Autodesk Inventor part; units mm, degrees
ref_plane "YZ Plane" through (0, 0, 0) normal (1, 0, 0) x (0, 1, 0)
ref_plane "XZ Plane" through (0, 0, 0) normal (0, 1, 0) x (-1, 0, 0)
ref_plane "XY Plane" through (0, 0, 0) normal (0, 0, 1) x (1, 0, 0)
sketch "Sketch1" plane through (0, 0, 0) normal (0, 0, 1) x (1, 0, 0)
  line L0 (0, 0) -> (298.0905, 0) construction
  line L1 (381, 254) -> (0, 254)
  line L2 (0, 254) -> (0, 0) construction
  line L3 (0, 254) -> (0, 0) construction
  line L4 (381, 254) -> (381, 177.8)
  line L5 (381, 177.8) -> (298.0905, 0)
  line L6 (0, 254) -> (0, 177.8)
  line L7 (82.9095, 0) -> (0, 177.8)
  line L8 (82.9095, 0) -> (298.0905, 0)
  dimension "d42" = 254
  dimension "d79" = 381
  dimension "d97" = 65
  dimension "d98" = 76.2
  dimension "d99" = 25
extrude "Plate1" add sketch "Sketch1" along normal blind 9.525
fillet "Corner Round1" radius 12.7 2 edges at (298.0905, 0, 4.7625) (82.9095, 0, 4.7625)
ref_plane "Work Plane1" through (0, 177.8, -13.208) normal (0, 1, 0) x (1, 0, 0)
sketch "Sketch10" plane through (0, 177.8, 9.525) normal (0, 0, 1) x (1, 0, 0)
  line L0 (342.9, 53.975) -> (342.9, 47.625) construction
  line L1 (333.375, 53.975) -> (333.375, 47.625)
  line L2 (352.425, 47.625) -> (352.425, 53.975)
  arc A0 (352.425, 53.975) -> (333.375, 53.975) centre (342.9, 53.975) ccw
  arc A1 (333.375, 47.625) -> (352.425, 47.625) centre (342.9, 47.625) ccw
  line L3 (50.8, 53.975) -> (50.8, 47.625) construction
  line L4 (41.275, 53.975) -> (41.275, 47.625)
  line L5 (60.325, 47.625) -> (60.325, 53.975)
  arc A2 (60.325, 53.975) -> (41.275, 53.975) centre (50.8, 53.975) ccw
  arc A3 (41.275, 47.625) -> (60.325, 47.625) centre (50.8, 47.625) ccw
  line L6 (0, 76.2) -> (381, 76.2)
  line L7 (381, 76.2) -> (381, 0)
  arc A4 (282.575, 47.625) -> (301.625, 47.625) centre (292.1, 47.625) ccw
  line L8 (282.575, 53.975) -> (282.575, 47.625)
  arc A5 (301.625, 53.975) -> (282.575, 53.975) centre (292.1, 53.975) ccw
  line L9 (301.625, 47.625) -> (301.625, 53.975)
  arc A6 (187.325, 53.975) -> (168.275, 53.975) centre (177.8, 53.975) ccw
  line L10 (187.325, 47.625) -> (187.325, 53.975)
  arc A7 (168.275, 47.625) -> (187.325, 47.625) centre (177.8, 47.625) ccw
  line L11 (168.275, 53.975) -> (168.275, 47.625)
  line L12 (0, 0) -> (0, 76.2)
  point P0 (342.9, 50.8)
  point P1 (50.8, 50.8)
  point P2 (41.275, 50.8)
  point P3 (168.275, 50.8)
  dimension "d83" = 19.05
  dimension "d85" = 6.35
  dimension "d100" = 25.4
  dimension "d101" = 38.1
  dimension "d104" = 50.8
  dimension "d111" = 127
  dimension "d116" = 50.8
extrude "Cut4" cut sketch "Sketch10" against normal blind 9.525
sketch "Sketch11" plane through (0, 0, 9.525) normal (0, 0, 1) x (1, 0, 0)
  line L0 (165.1, 127) -> (241.3, 127)
  line L1 (254, 114.3) -> (254, 38.1)
  line L2 (241.3, 25.4) -> (165.1, 25.4)
  line L3 (152.4, 38.1) -> (152.4, 114.3)
  line L4 (152.4, 127) -> (254, 25.4) construction
  line L5 (254, 127) -> (152.4, 25.4) construction
  arc A0 (254, 114.3) -> (241.3, 127) centre (241.3, 114.3) ccw
  arc A1 (165.1, 127) -> (152.4, 114.3) centre (165.1, 114.3) ccw
  arc A2 (152.4, 38.1) -> (165.1, 25.4) centre (165.1, 38.1) ccw
  arc A3 (241.3, 25.4) -> (254, 38.1) centre (241.3, 38.1) ccw
  line L6 (289.9997, 0) -> (0, 0)
  line L7 (0, 0) -> (0, 254)
  point P0 (203.2, 76.2)
  point P1 (12.7, 0)
  point P2 (0, 12.7)
  point P3 (0, 155.067)
  dimension "d90" = 101.6
  dimension "d91" = 101.6
  dimension "d92" = 12.7
  dimension "d93" = 25.4
  dimension "d94" = 152.4
extrude "Cut5" cut sketch "Sketch11" against normal blind 9.525
fillet "Corner Round4" radius 6.35 4 edges at (381, 254, 4.7625) (381, 177.8, 4.7625) (0, 254, 4.7625) (0, 177.8, 4.7625)
equation "\"d88\" = Thickness"
equation "\"d95\" = Thickness"
equation "\"d15\" = Thickness"
equation "\"BendReliefWidth\" = Thickness"
equation "\"BendReliefDepth\" = 0.5 * Thickness"
equation "\"CornerReliefSize\" = 4 * Thickness"
equation "\"MinimumRemnant\" = 2 * Thickness"
equation "\"TransitionRadius\" = BendRadius"
equation "\"JacobiRadiusSize\" = Thickness"
equation "\"GapSize\" = Thickness"
properties part number "Front Hitch Model-1_Sheet-RH" material "SS304"
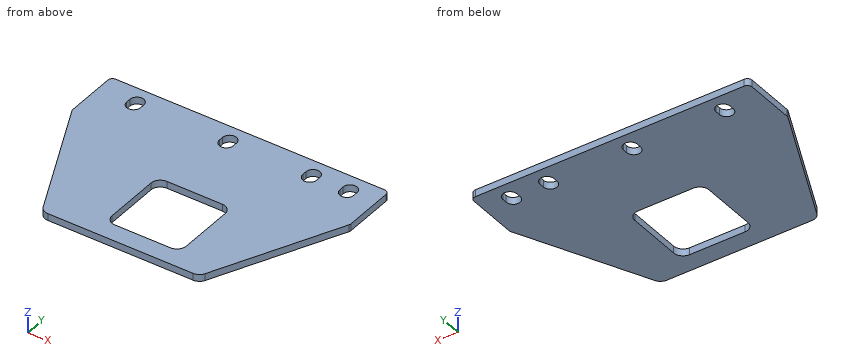
For this review, take the finished solid that the model builds, in its own axes (mm). Round coordinates to 2 decimals unless told otherwise and drop trailing zeros. Order: outer loops, then holes, each group sorted by start corner. A loop starts at its lowest first (then second) coordinate and runs counter-clockwise, first axis right, second up. Notation, with made-up numbers: (-29.5, 77) -> (-10.5, 77) arc R23 cw to (-10.5, 90) -> close; hole circle Ø11 at (26, 29). An arc over 180 degrees is marked (long way). Put each result on its own line as item: value.
Q1. Add section D-D on z = 2. State how many separate pieces and enclosed holes the cut face has, plus the area to 3 significant figures.
Check result:
separate pieces: 1
enclosed holes: 5
area: 70,200 mm2
Q2. Add section B-B on x = 177.8. Write out the cut boundary in (y, z) (3 decimals).
Check result:
outline: (0, 0) -> (25.4, 0) -> (25.4, 9.525) -> (0, 9.525) -> close; (127, 0) -> (215.9, 0) -> (215.9, 9.525) -> (127, 9.525) -> close; (241.3, 0) -> (254, 0) -> (254, 9.525) -> (241.3, 9.525) -> close
Q3. For probe 1 along Y at (x, z) = (200, 8.5); probe 2 along Y at (x, z) = (172.5, 2); probe 3 along X at (y, z) = (221, 0.75), list the stretches that pass through material, from the lowest coordinate up. Write a range as [from, to].
Check result:
probe 1: [0, 25.4], [127, 254]
probe 2: [0, 25.4], [127, 217.51], [239.69, 254]
probe 3: [0, 42.37], [59.23, 169.37], [186.23, 283.67], [300.53, 334.47], [351.33, 381]
Q4. Add section A-A on x = 223. Write out the cut boundary in (y, z) (3 decimals), plus the area to 3 significant figures.
Check result:
outline: (0, 0) -> (25.4, 0) -> (25.4, 9.525) -> (0, 9.525) -> close; (127, 0) -> (254, 0) -> (254, 9.525) -> (127, 9.525) -> close
area: 1,450 mm2
Q5. Insertion check: pin 1 Ø2 at (y, z) = (89, 4.5) entering from +X; pin 2 Ø8 at (x, y) = (340, 111.5) entering from -Z; pin 3 Ø3 at (y, z) = (91, 4) entering from -X; pin 4 Ø3 at (y, z) = (142, 7) entering from -X. Each pin has a flat end and moves straight along its axis. Give the tip position at first contact, or say it passes through.
Check result:
pin 1: x = 340.06
pin 2: z = 0
pin 3: x = 39.78
pin 4: x = 15.99
Q6. Add section C-C on y = 79. Write out the cut boundary in (x, z) (3 decimals).
Check result:
outline: (46.071, 0) -> (152.4, 0) -> (152.4, 9.525) -> (46.071, 9.525) -> close; (254, 0) -> (334.929, 0) -> (334.929, 9.525) -> (254, 9.525) -> close
